Autodesk Inventor part; units mm, degrees
ref_plane "YZ Plane" through (0, 0, 0) normal (1, 0, 0) x (0, 1, 0)
ref_plane "XZ Plane" through (0, 0, 0) normal (0, 1, 0) x (-1, 0, 0)
ref_plane "XY Plane" through (0, 0, 0) normal (0, 0, 1) x (1, 0, 0)
sketch "Sketch1" plane through (0, 0, 0) normal (0, 0, 1) x (1, 0, 0)
  line L0 (-13, -16.25) -> (13, -16.25)
  line L1 (13, -16.25) -> (13, 16.25)
  line L2 (13, 16.25) -> (-13, 16.25)
  line L3 (-13, 16.25) -> (-13, -16.25)
  line L4 (-13, -16.25) -> (13, 16.25) construction
  line L5 (13, -16.25) -> (-13, 16.25) construction
  line L6 (-10.5, 1.5) -> (10.5, 1.5) construction
  line L7 (10.5, 1.5) -> (10.5, 14) construction
  line L8 (10.5, 14) -> (-10.5, 14) construction
  line L9 (-10.5, 14) -> (-10.5, 1.5) construction
  line L10 (-10.5, 1.5) -> (10.5, 14) construction
  line L11 (10.5, 1.5) -> (-10.5, 14) construction
  circle A0 centre (-10.5, 14) radius 1.15
  circle A1 centre (10.5, 14) radius 1.15
  circle A2 centre (10.5, 1.5) radius 1.15
  circle A3 centre (-10.5, 1.5) radius 1.15
  line L12 (-13, -11.25) -> (-4, -11.25) construction
  line L13 (-4, -11.25) -> (-4, -16.25)
  line L14 (-4, -16.25) -> (-13, -16.25)
  line L15 (-13, -16.25) -> (-13, -11.25)
  line L16 (-13, -11.25) -> (-4, -16.25) construction
  line L17 (-4, -11.25) -> (-13, -16.25) construction
  line L18 (4, -11.25) -> (13, -11.25) construction
  line L19 (13, -11.25) -> (13, -16.25)
  line L20 (13, -16.25) -> (4, -16.25)
  line L21 (4, -16.25) -> (4, -11.25)
  line L22 (4, -11.25) -> (13, -16.25) construction
  line L23 (13, -11.25) -> (4, -16.25) construction
  line L24 (-4, -11.25) -> (4, -11.25)
  line L25 (-2.6, -8.85) -> (2.6, -8.85)
  line L26 (2.6, -8.85) -> (2.6, -3.65)
  line L27 (2.6, -3.65) -> (-2.6, -3.65)
  line L28 (-2.6, -3.65) -> (-2.6, -8.85)
  line L29 (-2.6, -8.85) -> (2.6, -3.65) construction
  line L30 (2.6, -8.85) -> (-2.6, -3.65) construction
  point P0 (0, 0)
  point P1 (0, 7.75)
  point P2 (0, 7.75)
  point P3 (-8.5, -13.75)
  point P4 (8.5, -13.75)
  point P5 (0, -11.25)
  point P6 (0, -16.25)
  point P7 (4, -16.25)
  point P8 (0, -6.25)
  dimension "d0" = 12.5
  dimension "d1" = 21
  dimension "d2" = 2.3
  dimension "d3" = 2.3
  dimension "d4" = 2.3
  dimension "d5" = 2.3
  dimension "d6" = 26
  dimension "d7" = 32.5
  dimension "d9" = 5
  dimension "d10" = 9
  dimension "d11" = 5
  dimension "d12" = 9
  dimension "d17" = 5.2
  dimension "d18" = 5.2
  dimension "d19" = 10
  dimension "d20" = 8.5
extrude "Extrusion1" add sketch "Sketch1" along normal blind 5 contours L3 L2 L1 L0 L21 L24 L13
chamfer "Chamfer1" distance 1.5 angle 45 2 edges at (13, 16.25, 2.5) (-13, 16.25, 2.5)
equation "\"d2\" = d3"
equation "\"d4\" = d2"
equation "\"d5\" = d4"
equation "\"d11\" = d9"
equation "\"d12\" = d10"
properties part number "camera-bracket"
Work out the finished part from the listing and answer in its coordinate system (mm). A direction names the side the tool comes from. Round coordinates to 2 decimals unless told otherwise and drop trailing zeros. Loops run counter-clockwise (first coordinate to the right, second up) from the corner with the lowest first, then second, coordinate; pieces in that order, holes last. Notation, with made-up numbers: (29, -0.5) -> (63, -0.5) arc R22 cw to (63, 17.5) -> close; hole circle Ø5 at (-35, -27). An arc over 180 degrees is marked (long way). Write each question's results on one line, items separated by ' | '. Start each with the question number.
1. Find the intervals of material crossed by probe 1 along Y at (x, z) = (-10.5, 3.2); probe 2 along X at (y, z) = (-4, 2.65); probe 3 along Y at (x, z) = (-1.5, 4.65), in increasing order. Write a range as from..to.
2. Section A-A (x = 0) is taken. Determine the outline of the cut face in (y, z).
3. Given pin 1 Ø1.5 at (x, y) = (-1.5, -6) entering from +Z; pin 2 Ø1.5 at (x, z) = (-0.5, 2) entering from -Y; pin 3 Ø3 at (x, y) = (1.5, -6.5) entering from -Z, each flat-ended and moving along its own axis, determine where each tip first touches the part or whether it passes through.
4. For a pull along Y with two mould halves and no side action, classify faces 4 (the face through (0, 16.25, 2)), 5 (the face through (-9.438, 14.44, 2.465)), 6 (the face through (0, 0, 5)) as +Y half, -Y half, draft (parallel to the pull), parting line (faces both ways), or undercut.
5. A tool of negligible diameter and unlimited length cuts with its end or side. For faces 1 (the face through (13, -1, 2)), 2 (the face through (-4, -14, 2)), 3 (the face through (0, -8.85, 2)), from which of +Z, -Z, +X, -X, +Y, -Y can it reach the whole face along a straight path? Write none if from no direction.
6. Section C-C (z = 3.85) is taken. Determine the outline of the cut face in (x, y).
7. Section D-D (x = 10.5) is taken. Determine the outline of the cut face in (y, z).
8. Section B-B (y = 14) is taken. Determine the outline of the cut face in (x, z), plus the area to 3 significant figures.
Evaluation:
1) probe 1: y = -16.25..0.35, 2.65..12.85, 15.15..16.25 | probe 2: x = -13..-2.6, 2.6..13 | probe 3: y = -11.25..-8.85, -3.65..16.25
2) outline: (-11.25, 0) -> (-8.85, 0) -> (-8.85, 5) -> (-11.25, 5) -> close; (-3.65, 0) -> (16.25, 0) -> (16.25, 5) -> (-3.65, 5) -> close
3) pin 1: passes through | pin 2: stops at y = -11.25 | pin 3: stops at z = 0
4) face 4: +Y half | face 5: undercut | face 6: draft
5) face 1: +Z, -Z, +X, +Y, -Y | face 2: +Z, -Z, -Y | face 3: +Z, -Z
6) outline: (-13, -16.25) -> (-4, -16.25) -> (-4, -11.25) -> (4, -11.25) -> (4, -16.25) -> (13, -16.25) -> (13, 14.75) -> (11.5, 16.25) -> (-11.5, 16.25) -> (-13, 14.75) -> close; hole circle Ø2.3 at (-10.5, 1.5); hole circle Ø2.3 at (-10.5, 14); hole (-2.6, -8.85) -> (2.6, -8.85) -> (2.6, -3.65) -> (-2.6, -3.65) -> close; hole circle Ø2.3 at (10.5, 1.5); hole circle Ø2.3 at (10.5, 14)
7) outline: (-16.25, 0) -> (0.35, 0) -> (0.35, 5) -> (-16.25, 5) -> close; (2.65, 0) -> (12.85, 0) -> (12.85, 5) -> (2.65, 5) -> close; (15.15, 0) -> (16.25, 0) -> (16.25, 5) -> (15.15, 5) -> close
8) outline: (-13, 0) -> (-11.65, 0) -> (-11.65, 5) -> (-13, 5) -> close; (-9.35, 0) -> (9.35, 0) -> (9.35, 5) -> (-9.35, 5) -> close; (11.65, 0) -> (13, 0) -> (13, 5) -> (11.65, 5) -> close | area: 107 mm2
